For this review, take the finished solid that the model builds, in its own axes (mm). Coordinates: 2 decimals unless noted, no trailing zeros. Loops run counter-clockwise (first coordinate to the right, second up) from the corner with the lowest first, then second, coordinate; pieces in that order, holes last. Notation, with made-up numbers: (72.25, 59) - (104.25, 59) arc R22 ccw to (104.25, 69) - close; hole circle Ø8 at (-26, -29.75). An arc over 180 degrees is marked (long way). Answer as a JSON object with one key per item and string values. Group by question number.
Item 1: To check wall thickness, follow line 1 (X direction, y = -100, z = -1.3); line 2 (Y direction, x = 20, z = -0.7); line 3 (X direction, y = -20, z = -0.6). State the ranges of each line that lie inside material, in increasing order.
Item 2: We need section A-A (y = -100). Give the boundary of the cut face in (x, z).
Item 3: Clearance check with flat-ended pins moving along their axes: pin 1 (5.5 mm diameter, centred on x = 20, y = -20, fed in from -Z); pin 2 (11.5 mm diameter, centred on x = 20, y = -100, fed in from -Z); pin 3 (1 mm diameter, centred on y = -32.5, z = -1.5, fed in from +X). State where each tip first meets the part, or that it passes through.
Item 4: We need section B-B (x = 20). Give the boundary of the cut face in (y, z), then the cut area to 3 significant figures.
Item 5: We need section C-C (z = -0.3). Give the boundary of the cut face in (x, y), then the cut area to 3 significant figures.
Item 6: We need section D-D (y = -60). Give the boundary of the cut face in (x, z).
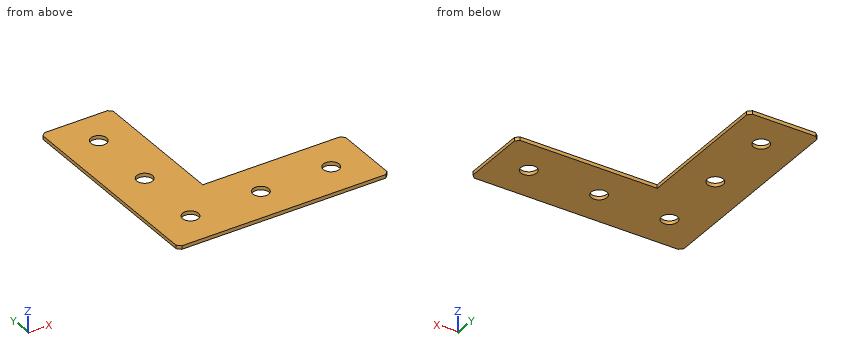
from build123d import *

# Parameters (mm, degrees)
EXTRUDE_1_DEPTH   = 2
HOLE_WIZARD_M81_D = 9
CHAMFER_1_SIZE    = 2


with BuildPart() as part:
    # Эскиз1 → Бобышка-Вытянуть1 (new body)
    with BuildSketch(Plane(origin=(0, 0, 0), x_dir=(1, 0, 0), z_dir=(0, 0, -1))):
        Polygon((0, 0), (0, 120), (120, 120), (120, 80), (40, 80), (40, 0), align=None)
    extrude(amount=EXTRUDE_1_DEPTH)

    # Отверстие с зазором M81 (through all)
    with Locations(Plane(origin=(0, 0, -2), x_dir=(1, 0, 0), z_dir=(0, 0, -1))):
        with Locations((60, 100), (20, 100), (20, 60), (20, 20), (100, 100)):
            Hole(HOLE_WIZARD_M81_D / 2)

    # Фаска1
    chamfer_1_edges = [part.edges().sort_by_distance(p)[0] for p in [
        (0, 0, -1),
        (0, -120, -1),
        (120, -120, -1),
        (120, -80, -1),
        (40, 0, -1),
    ]]
    chamfer(chamfer_1_edges, length=CHAMFER_1_SIZE)


solid = part.part
Check sheet entries:
{
 "1": {"line 1": "x = 0 to 15.5, 24.5 to 55.5, 64.5 to 95.5, 104.5 to 120", "line 2": "y = -120 to -104.5, -95.5 to -64.5, -55.5 to -24.5, -15.5 to 0", "line 3": "x = 0 to 15.5, 24.5 to 40"},
 "2": {"outline": "(0, -2) - (15.5, -2) - (15.5, 0) - (0, 0) - close; (24.5, -2) - (55.5, -2) - (55.5, 0) - (24.5, 0) - close; (64.5, -2) - (95.5, -2) - (95.5, 0) - (64.5, 0) - close; (104.5, -2) - (120, -2) - (120, 0) - (104.5, 0) - close"},
 "3": {"pin 1": "passes through", "pin 2": "stops at z = -2", "pin 3": "stops at x = 40"},
 "4": {"outline": "(-120, -2) - (-104.5, -2) - (-104.5, 0) - (-120, 0) - close; (-95.5, -2) - (-64.5, -2) - (-64.5, 0) - (-95.5, 0) - close; (-55.5, -2) - (-24.5, -2) - (-24.5, 0) - (-55.5, 0) - close; (-15.5, -2) - (0, -2) - (0, 0) - (-15.5, 0) - close", "area": "186 mm2"},
 "5": {"outline": "(0, -118) - (2, -120) - (118, -120) - (120, -118) - (120, -82) - (118, -80) - (40, -80) - (40, -2) - (38, 0) - (2, 0) - (0, -2) - close; hole circle Ø9 at (20, -100); hole circle Ø9 at (20, -60); hole circle Ø9 at (20, -20); hole circle Ø9 at (60, -100); hole circle Ø9 at (100, -100)", "area": "7,670 mm2"},
 "6": {"outline": "(0, -2) - (15.5, -2) - (15.5, 0) - (0, 0) - close; (24.5, -2) - (40, -2) - (40, 0) - (24.5, 0) - close"}
}
